The listing builds one solid part. Answer for the finished solid, in the listing's coordinates (mm). A direction names the side the tool comes from. Coordinates: 2 decimals unless noted, no trailing zeros. Loops run counter-clockwise (first coordinate to the right, second up) from the corner with the lowest first, then second, coordinate; pieces in that order, holes last. Notation, with made-up numbers: M 61.5,16.25 L 107.5,16.25 A8 ccw 107.5,21.25 Z; hole C 77.5,88.5 d8. An arc over 180 degrees is marked long. Return JSON: item names as keys, results as strings. Group by question number.
1. Section D-D (y = -11.5) is taken. Write down the section's boundary in (x, z), then the cut area to 3 significant figures.
2. Section A-A (y = 7.5) is taken. Write down the section's boundary in (x, z).
3. Section C-C (x = 171.5) is taken. Write down the section's boundary in (y, z).
4. Section B-B (z = -8) is taken. Write down the section's boundary in (x, y), then the cut area to 3 significant figures.
5. The mould has two halves that part along X. Classify faces 3 (the face through (220, -14, 2)), 4 (the face through (91.983, -14.24, -12.76)), 5 (the face through (108, 0, 18)), 6 (the face through (213.002, -7.412, 19.014)): pulls with the +X half, pulls with the -X half, needs draft (parallel to the pull), parting line crosses it, or undercut.
6. Which of the six approach directions +Z, -Z, +X, -X, +Y, -Y give full straight-line access (tool end or side, diameter ignored) to faces 1 (the face through (181.002, -7.412, -18.986)), 2 (the face through (108, 13.5, 0))?
7. Straight lines are drawn through the part: L1, parallel to Z at x = 210, y = 14.35; L2, parallel to Y at x = 215, z = -18.75; L3, parallel to Z at x = 75.5, y = -11.5. For each, find the intervals that lie inside material, in ascending order. Write a range as from..to.
```python
from build123d import *

# Parameters (mm, degrees)
SKETCH_1_W          = 40
SKETCH_1_H          = 30
SKETCH_1_W_2        = 36
SKETCH_1_H_2        = 27
EXTRUDE_1_DEPTH     = 220
SKETCH_2_R          = 2
CUT_EXTRUDE_1_DEPTH = 223.934968096
SKETCH_3_R          = 2
CUT_EXTRUDE_2_DEPTH = 223.934968096
SKETCH_4_R          = 2
CUT_EXTRUDE_3_DEPTH = 225.10934831


with BuildPart() as part:
    # 草图1 → 凸台-拉伸1 (new body)
    with BuildSketch(Plane(origin=(0, 0, 0), x_dir=(0, 0, -1), z_dir=(1, 0, 0))):
        Rectangle(SKETCH_1_W, SKETCH_1_H)
        Rectangle(SKETCH_1_W_2, SKETCH_1_H_2, mode=Mode.SUBTRACT)
    extrude(amount=EXTRUDE_1_DEPTH)

    # 草图2 → 切除-拉伸1 (cut, through all)
    with BuildSketch(Plane(origin=(0, 15, 0), x_dir=(1, 0, 0), z_dir=(0, 1, 0))):
        with Locations(Location((210, -7, 0), (0, 0, 270))):
            Circle(SKETCH_2_R)
        with Locations(Location((210, 13, 0), (0, 0, 270))):
            Circle(SKETCH_2_R)
        with Locations(Location((188, 13, 0), (0, 0, 270))):
            Circle(SKETCH_2_R)
        with Locations(Location((188, -7, 0), (0, 0, 270))):
            Circle(SKETCH_2_R)
    extrude(amount=-CUT_EXTRUDE_1_DEPTH, mode=Mode.SUBTRACT)

    # 草图3 → 切除-拉伸2 (cut, through all)
    with BuildSketch(Plane(origin=(0, 15, 0), x_dir=(1, 0, 0), z_dir=(0, 1, 0))):
        with Locations(Location((90, 12.5, 0), (0, 0, 270))):
            Circle(SKETCH_3_R)
        with Locations(Location((110, 12.5, 0), (0, 0, 270))):
            Circle(SKETCH_3_R)
        with Locations(Location((110, -12.5, 0), (0, 0, 270))):
            Circle(SKETCH_3_R)
        with Locations(Location((90, -12.5, 0), (0, 0, 270))):
            Circle(SKETCH_3_R)
    extrude(amount=-CUT_EXTRUDE_2_DEPTH, mode=Mode.SUBTRACT)

    # 草图4 → 切除-拉伸3 (cut, through all)
    with BuildSketch(Plane.XY.offset(20)):
        with Locations((183, 7.5)):
            Circle(SKETCH_4_R)
        with Locations((215, 7.5)):
            Circle(SKETCH_4_R)
        with Locations((215, -7.5)):
            Circle(SKETCH_4_R)
        with Locations((183, -7.5)):
            Circle(SKETCH_4_R)
    extrude(amount=-CUT_EXTRUDE_3_DEPTH, mode=Mode.SUBTRACT)


solid = part.part
```
Worked out:
{
 "1": {"outline": "M 0,-20 L 220,-20 L 220,-18 L 0,-18 Z; M 0,18 L 220,18 L 220,20 L 0,20 Z", "area": "880 mm^2"},
 "2": {"outline": "M 0,-20 L 181,-20 L 181,-18 L 0,-18 Z; M 0,18 L 181,18 L 181,20 L 0,20 Z; M 185,-20 L 213,-20 L 213,-18 L 185,-18 Z; M 185,18 L 213,18 L 213,20 L 185,20 Z; M 217,-20 L 220,-20 L 220,-18 L 217,-18 Z; M 217,18 L 220,18 L 220,20 L 217,20 Z"},
 "3": {"outline": "M -15,-20 L 15,-20 L 15,20 L -15,20 Z; hole M -13.5,-18 L 13.5,-18 L 13.5,18 L -13.5,18 Z"},
 "4": {"outline": "M 0,-15 L 220,-15 L 220,-13.5 L 0,-13.5 Z; M 0,13.5 L 220,13.5 L 220,15 L 0,15 Z", "area": "660 mm^2"},
 "5": {"face 3": "pulls with the +X half", "face 4": "undercut", "face 5": "needs draft", "face 6": "undercut"},
 "6": {"face 1": "+Z, -Z", "face 2": "+X, -X"},
 "7": {"L1": "-20..-15, -11..5, 9..20", "L2": "-15..-9.5, -5.5..5.5, 9.5..15", "L3": "-20..-18, 18..20"}
}
